Could you check a few things on this model? Use its own coordinates, in mm. Give positions to 0.01 mm unless a question says otherwise; leave off trailing zeros. Order: outer loops, then holes, each group sorted by start corner. A loop starts at its lowest first (then second) coordinate and runs counter-clockwise, first axis right, second up. Notation, with made-up numbers: (9.25, 60) -> (51.25, 60) arc R25 ccw to (51.25, 80) -> close; hole circle Ø9 at (12.25, 61). An arc over 180 degrees is marked (long way). Write each question's results on one line, items separated by ' | '.
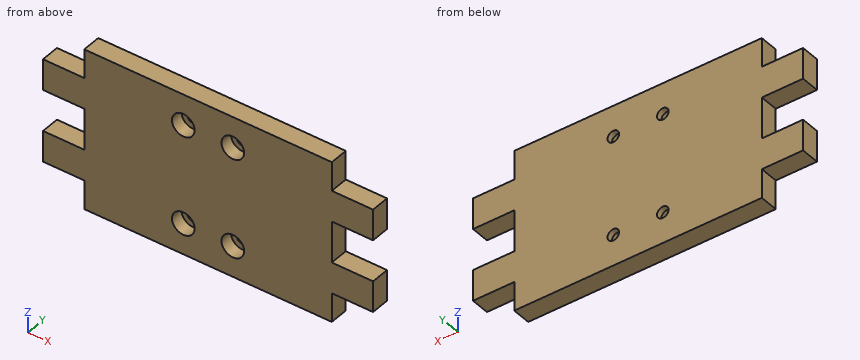
```python
from build123d import *

# Parameters (mm, degrees)
SKETCH1_W                       = 25
SKETCH1_H                       = 4.5
BOSS_EXTRUDE1_DEPTH             = 30
SKETCH2_W                       = 7.5
SKETCH2_H                       = 4.5
BOSS_EXTRUDE2_DEPTH             = 10
ESQUISSE1_W                     = 60
ESQUISSE1_H                     = 4.5
BOSS_EXTRU_1_DEPTH              = 7
CBORE_FOR_M3_SBHCS2_D           = 2.8
CBORE_FOR_M3_SBHCS2_CBORE_D     = 5.5
CBORE_FOR_M3_SBHCS2_CBORE_DEPTH = 3.1


with BuildPart() as part:
    # Sketch1 → Boss-Extrude1 (new, symmetric)
    with BuildSketch(Plane(origin=(0, 0, 0), x_dir=(0, 0, -1), z_dir=(1, 0, 0))):
        Rectangle(SKETCH1_W, SKETCH1_H)
    extrude(amount=BOSS_EXTRUDE1_DEPTH, both=True)

    # Sketch2 → Boss-Extrude2 (add)
    with BuildSketch(Plane(origin=(30, 0, 0), x_dir=(0, 0, -1), z_dir=(1, 0, 0))):
        with Locations((-8.75, 0)):
            Rectangle(SKETCH2_W, SKETCH2_H)
        with Locations((8.75, 0)):
            Rectangle(SKETCH2_W, SKETCH2_H)
    boss_extrude2 = extrude(amount=BOSS_EXTRUDE2_DEPTH)

    # Esquisse1 → Boss.-Extru.1 (add)
    with BuildSketch(Plane.XY.offset(12.5)):
        Rectangle(ESQUISSE1_W, ESQUISSE1_H)
    boss_extru_1 = extrude(amount=BOSS_EXTRU_1_DEPTH)

    # Symétrie1: Boss.-Extru.1 across plane
    add(boss_extru_1.mirror(Plane.XY))

    # Mirror1: Boss-Extrude2 across plane
    add(boss_extrude2.mirror(Plane(origin=(0, 0, 0), x_dir=(0, 0, 1), z_dir=(1, 0, 0))))

    # CBORE for M3 SBHCS2 (through all)
    with Locations(Plane(origin=(0, -2.25, 0), x_dir=(-1, 0, 0), z_dir=(0, -1, 0))):
        with Locations((-6, 12), (6, 12), (6, -12), (-6, -12)):
            CounterBoreHole(CBORE_FOR_M3_SBHCS2_D / 2, CBORE_FOR_M3_SBHCS2_CBORE_D / 2, CBORE_FOR_M3_SBHCS2_CBORE_DEPTH)


solid = part.part
```
Q1. I need wall thicknesses on line 1 along Z through (x, y) = (6, -1.15); line 2 along X through (y, z) = (-0.1, 12); line 3 along Z through (x, y) = (6, 1.7). Which ranges of each line are inside material? Lowest first, please.
Here are the results:
line 1: z = -19.5 to -14.75, -9.25 to 9.25, 14.75 to 19.5 | line 2: x = -40 to -8.75, -3.25 to 3.25, 8.75 to 40 | line 3: z = -19.5 to -13.4, -10.6 to 10.6, 13.4 to 19.5
Q2. I'm going to push flat-ended pins straight in: pin 1 Ø1.3 at (y, z) = (0, -17) entering from -X; pin 2 Ø1.3 at (y, z) = (1, -14.5) entering from +X; pin 3 Ø3.5 at (x, z) = (6, -12) entering from -Y. Where does each tip first touch, or does it pass through?
Here are the results:
pin 1: stops at x = -30 | pin 2: stops at x = 30 | pin 3: stops at y = 0.85
Q3. Suppose I cut it at B-B on y = -0.4. Please give me the cut outline in (x, z).
Here are the results:
outline: (-40, -12.5) -> (-30, -12.5) -> (-30, -19.5) -> (30, -19.5) -> (30, -12.5) -> (40, -12.5) -> (40, -5) -> (30, -5) -> (30, 5) -> (40, 5) -> (40, 12.5) -> (30, 12.5) -> (30, 19.5) -> (-30, 19.5) -> (-30, 12.5) -> (-40, 12.5) -> (-40, 5) -> (-30, 5) -> (-30, -5) -> (-40, -5) -> close; hole circle Ø5.5 at (-6, -12); hole circle Ø5.5 at (-6, 12); hole circle Ø5.5 at (6, -12); hole circle Ø5.5 at (6, 12)
Q4. Suppose I cut it at A-A on x = -6. Please give me the cut outline in (y, z).
Here are the results:
outline: (-2.25, -19.5) -> (2.25, -19.5) -> (2.25, -13.4) -> (0.85, -13.4) -> (0.85, -14.75) -> (-2.25, -14.75) -> close; (-2.25, -9.25) -> (0.85, -9.25) -> (0.85, -10.6) -> (2.25, -10.6) -> (2.25, 10.6) -> (0.85, 10.6) -> (0.85, 9.25) -> (-2.25, 9.25) -> close; (-2.25, 14.75) -> (0.85, 14.75) -> (0.85, 13.4) -> (2.25, 13.4) -> (2.25, 19.5) -> (-2.25, 19.5) -> close
